For this review, take the finished solid that the model builds, in its own axes (mm). A direction names the side the tool comes from. Round coordinates to 2 decimals unless told otherwise and drop trailing zeros. Write each loop counter-clockwise with the first axis right and the second up, starting at its lowest first coordinate (ties: lowest second). Pieces come first, ordered by that corner, then holes. Notation, with made-up numbers: M 52.25,51 L 83.25,51 A26 cw 83.25,82 Z; hole C 41,-21.75 d3. An arc over 180 degrees is marked long. Use one line per item in the form item = value. Start each with the question number.
Item 1: For faces 1 (the flat face through (99, 5, -62)), 2 (the flat face through (99, 3, -24)), list the 3-axis set-ups (+Z, -Z, +X, -X, +Y, -Y) from which the entire face can be reached by the end or side of a thin tool; tool diameter is ignored.
Item 2: For line 1 (Z direction, x = 10, y = 2.6) (3 decimals); line 2 (Z direction, x = 190, y = 3.6) (3 decimals); line 3 (X direction, y = 3.45, z = -63) (3 decimals), list the stretches that pass through material, from the lowest coordinate up. Write a range as [from, to].
Item 3: Add section B-B (z = -36.5). State the section outline as (x, y) points, and give its area (3 significant figures).
Item 4: Add section A-A (y = 4.2). State the section outline as (x, z) points (3 decimals), and give its area (3 significant figures).
Item 5: Add section C-C (x = 100). State the section outline as (y, z) points, and give its area (3 significant figures).
Item 6: For P1, Ø2.5, axis at x = 109.5, z = -25, coming from the +Y side, flat-tipped, find the tip position at first contact; note if it passes through.
Item 7: Add section D-D (x = 10). State the section outline as (y, z) points (3 decimals), and give its area (4 significant figures).
from build123d import *

# Parameters (mm, degrees)
SKETCH1_W                   = 200
SKETCH1_H                   = 73
RIGHT_WALL_DEPTH            = 5
F_1_4_0_2500_DOWEL_HOLE1_D  = 6.35
TAP_DRILL_FOR_1_4_28_TAP2_D = 5.4102
SKETCH24_W                  = 200
SKETCH24_H                  = 5
CUT_EXTRUDE1_DEPTH          = 2


with BuildPart() as part:
    # Sketch1 → right wall (new body)
    with BuildSketch(Plane(origin=(0, 0, 0), x_dir=(1, 0, 0), z_dir=(0, 1, 0))):
        with Locations((100, 36.5)):
            Rectangle(SKETCH1_W, SKETCH1_H)
    extrude(amount=RIGHT_WALL_DEPTH)

    # 1/4 (0.2500) Dowel Hole1 (through all)
    with Locations(Plane(origin=(0, 0, 0), x_dir=(-1, 0, 0), z_dir=(0, -1, 0))):
        with Locations((-10, 10), (-10, 63), (-190, 63), (-190, 10)):
            Hole(F_1_4_0_2500_DOWEL_HOLE1_D / 2)

    # Tap Drill for 1/4-28 Tap2 (through all)
    with Locations(Plane(origin=(0, 0, 0), x_dir=(-1, 0, 0), z_dir=(0, -1, 0))):
        with Locations((-100, 36.5)):
            Hole(TAP_DRILL_FOR_1_4_28_TAP2_D / 2)

    # Sketch24 → Cut-Extrude1 (cut)
    with BuildSketch(Plane(origin=(0, 5, 0), x_dir=(1, 0, 0), z_dir=(0, 1, 0))):
        with Locations((100, 49)):
            Rectangle(SKETCH24_W, SKETCH24_H)
        with Locations((100, 24)):
            Rectangle(SKETCH24_W, SKETCH24_H)
    extrude(amount=-CUT_EXTRUDE1_DEPTH, mode=Mode.SUBTRACT)


solid = part.part
Calculated:
q1.face_1 = +Z, -Z, +X, -X, +Y
q1.face_2 = +X, -X, +Y
q2.line_1 = [-73, -66.175], [-59.825, -13.175], [-6.825, 0]
q2.line_2 = [-73, -66.175], [-59.825, -51.5], [-46.5, -26.5], [-21.5, -13.175], [-6.825, 0]
q2.line_3 = [0, 6.825], [13.175, 186.825], [193.175, 200]
q3.outline = M 0,0 L 97.29,0 L 97.29,5 L 0,5 Z; M 102.71,0 L 200,0 L 200,5 L 102.71,5 Z
q3.area = 973 mm^2
q4.outline = M 0,-73 L 200,-73 L 200,-51.5 L 0,-51.5 Z; M 0,-46.5 L 200,-46.5 L 200,-26.5 L 0,-26.5 Z; M 0,-21.5 L 200,-21.5 L 200,0 L 0,0 Z; hole C 10,-63 d6.35; hole C 10,-10 d6.35; hole C 100,-36.5 d5.41; hole C 190,-63 d6.35; hole C 190,-10 d6.35
q4.area = 12,500 mm^2
q5.outline = M 0,-73 L 5,-73 L 5,-51.5 L 3,-51.5 L 3,-46.5 L 5,-46.5 L 5,-39.21 L 0,-39.21 Z; M 0,-33.79 L 5,-33.79 L 5,-26.5 L 3,-26.5 L 3,-21.5 L 5,-21.5 L 5,0 L 0,0 Z
q5.area = 318 mm^2
q6.P1 = 3
q7.outline = M 0,-73 L 5,-73 L 5,-66.175 L 0,-66.175 Z; M 0,-59.825 L 5,-59.825 L 5,-51.5 L 3,-51.5 L 3,-46.5 L 5,-46.5 L 5,-26.5 L 3,-26.5 L 3,-21.5 L 5,-21.5 L 5,-13.175 L 0,-13.175 Z; M 0,-6.825 L 5,-6.825 L 5,0 L 0,0 Z
q7.area = 281.5 mm^2
